Could you check a few things on this drawing? It's one solid part, dimensions in mm from its lowest x, y, z. Round coordinates to 2 decimals unless told otherwise and drop trailing zeros. Write each loop counter-clockwise with the first axis right and the second up, starting at its lowest first coordinate (ties: lowest second). Pieces come first, ordered by that corner, then holes. Notation, with made-up numbers: (66.5, -15.5) - (97.5, -15.5) arc R18 ccw to (97.5, 14.5) - close; hole circle Ø7 at (36, -38). An arc over 180 degrees is marked (long way). One line per question, with ' | ' between items. Start each with the question number.
(1) Imagine slicing it at D-D (z = 12). Write out the boundary of the cut face in (x, y) (3 decimals).
(2) Imagine slicing it at C-C (z = 7.25). Write out the boundary of the cut face in (x, y) (3 decimals), plus the area to 3 significant figures.
(3) If I drill on L1, parallel to Y at x = 8, z = 6.35 (3 decimals), over which ranges is the centre line in solid material (lowest first)?
(4) Thinking about a two-plate mould opening in X: for the marked faces 1, 2, 3 and 4, which applies, pulls with the +X half, pulls with the -X half, needs draft (parallel to the pull), parting line crosses it, or undercut?
(5) Imagine slicing it at A-A (y = 6.35). Write out the boundary of the cut face in (x, z) (3 decimals), plus the area to 3 significant figures.
(6) Imagine slicing it at B-B (x = 3.5). Write out the boundary of the cut face in (y, z) (3 decimals).
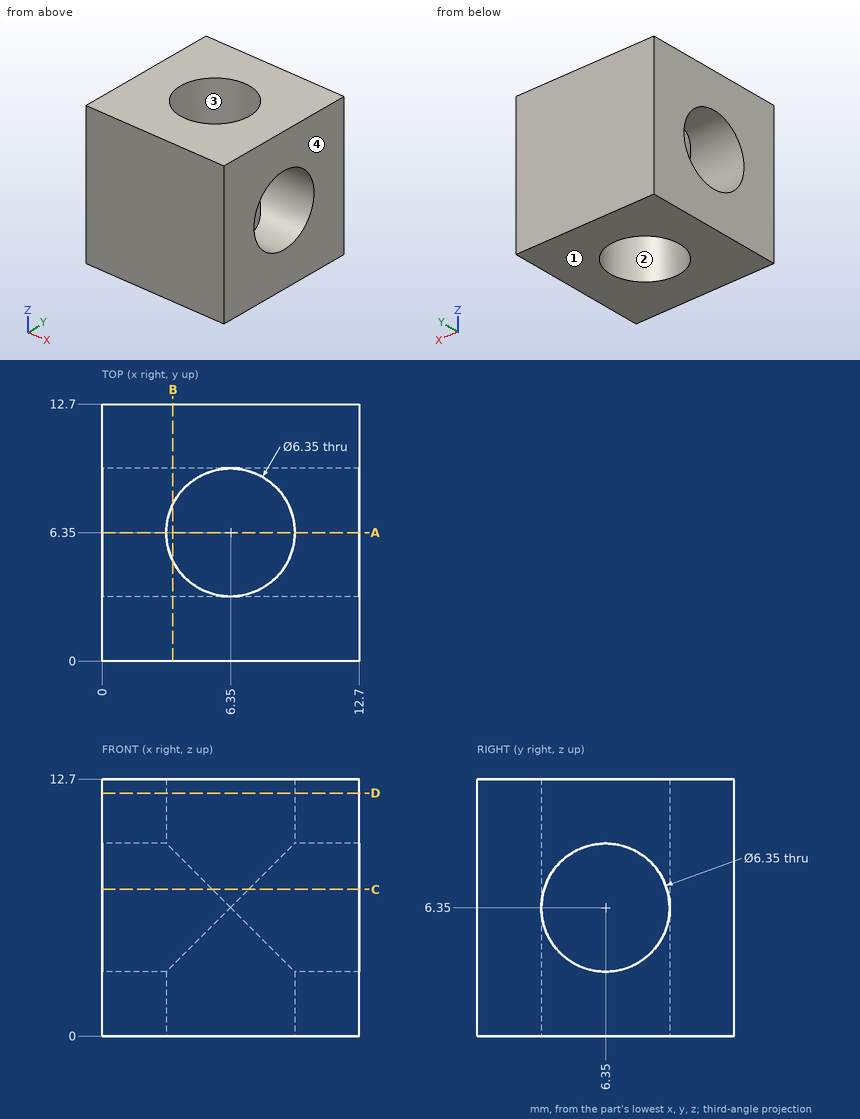
Check sheet entries:
1) outline: (0, 0) - (12.7, 0) - (12.7, 12.7) - (0, 12.7) - close; hole circle Ø6.35 at (6.35, 6.35)
2) outline: (0, 0) - (12.7, 0) - (12.7, 3.305) - (7.25, 3.305) arc R3.175 cw to (5.45, 3.305) - (0, 3.305) - close; (0, 9.395) - (5.45, 9.395) arc R3.175 cw to (7.25, 9.395) - (12.7, 9.395) - (12.7, 12.7) - (0, 12.7) - close | area: 83.6 mm^2
3) L1: 0 to 3.175, 9.525 to 12.7
4) face 1: needs draft | face 2: undercut | face 3: undercut | face 4: pulls with the +X half
5) outline: (0, 0) - (3.175, 0) - (3.175, 3.175) - (0, 3.175) - close; (0, 9.525) - (3.175, 9.525) - (3.175, 12.7) - (0, 12.7) - close; (9.525, 0) - (12.7, 0) - (12.7, 3.175) - (9.525, 3.175) - close; (9.525, 9.525) - (12.7, 9.525) - (12.7, 12.7) - (9.525, 12.7) - close | area: 40.3 mm^2
6) outline: (0, 0) - (4.951, 0) - (4.951, 3.5) arc R3.175 cw to (4.951, 9.2) - (4.951, 12.7) - (0, 12.7) - close; (7.749, 0) - (12.7, 0) - (12.7, 12.7) - (7.749, 12.7) - (7.749, 9.2) arc R3.175 cw to (7.749, 3.5) - close
